The model under review builds one solid part; all positions refer to its coordinate system, in mm. A direction names the side the tool comes from. Coordinates: 2 decimals unless noted, no trailing zeros. Order: outer loops, then holes, each group sorted by start corner. A loop starts at its lowest first (then second) coordinate and runs counter-clockwise, first axis right, second up. Notation, with made-up numbers: (45.25, -2) - (72.25, -2) arc R7 cw to (72.25, 8) - close; hole circle Ø9 at (22, 42). An arc over 180 degrees is marked (long way). Answer in a Markdown table with one row per item.
```python
from build123d import *

# Parameters (mm, degrees)
F0_W     = 1620
F0_H     = 1350
F1_DEPTH = 525
F2_W     = 630
F2_H     = 540
F3_DEPTH = 420
F4_W     = 990
F4_H     = 450
F5_DEPTH = 540
F7_DEPTH = 1620.001
F9_DEPTH = 1050.001


with BuildPart() as f1:
    # F0 (on Front) → F1 (new body, symmetric)
    with BuildSketch(Plane.XZ):
        Rectangle(F0_W, F0_H)
    extrude(amount=F1_DEPTH, both=True)

    # F2 (on face) → F3 (cut)
    with BuildSketch(Plane.XZ.offset(525)):
        with Locations((-495, -405)):
            Rectangle(F2_W, F2_H)
        with Locations((495, -405)):
            Rectangle(F2_W, F2_H)
    extrude(amount=-F3_DEPTH, mode=Mode.SUBTRACT)

    # F4 (on face) → F5 (cut)
    with BuildSketch(Plane.XY.offset(675)):
        with Locations((-315, -300)):
            Rectangle(F4_W, F4_H)
    extrude(amount=-F5_DEPTH, mode=Mode.SUBTRACT)

    # F6 (on face) → F7 (cut, through all)
    with BuildSketch(Plane.YZ.offset(810)):
        Polygon((135, 675), (-525, 675), (-525, 135), align=None)
    extrude(amount=-F7_DEPTH, mode=Mode.SUBTRACT)

    # F8 (on face) → F9 (cut, through all)
    with BuildSketch(Plane.XZ.offset(525)):
        Polygon((180, 675), (810, 135), (810, 675), align=None)
    extrude(amount=-F9_DEPTH, mode=Mode.SUBTRACT)


solid = f1.part
```
Item 1: To check wall thickness, follow line 1 (X direction, y = -370.5, z = -157); line 2 (Y direction, x = 679, z = -582); line 3 (Y direction, x = -382, z = 205.5). State the ranges of each line that lie inside material, in increasing order. Write a range as from..to.
Check values:
| item | result |
|---|---|
| line 1 | -180..180 |
| line 2 | -105..525 |
| line 3 | -75..525 |
Item 2: We need section D-D, the plane x = 18. Write out the cut boundary in (y, z).
Check values:
| item | result |
|---|---|
| outline | (-525, -675) - (525, -675) - (525, 675) - (135, 675) - (-75, 503.18) - (-75, 135) - (-525, 135) - close |
Item 3: Clearance check with flat-ended pins moving along their axes: pin 1 Ø12 at (y, z) = (144, 455.5) entering from +X; pin 2 Ø1.5 at (y, z) = (343, 179.5) entering from +X; pin 3 Ø1 at (y, z) = (-161, 209) entering from -X. State where each tip first meets the part, or that it passes through.
Check values:
| item | result |
|---|---|
| pin 1 | x = 443.08 |
| pin 2 | x = 758.96 |
| pin 3 | x = 180 |
Item 4: We need section C-C, the plane y = -396.5. Write out the cut boundary in (x, z), then the cut area to 3 significant figures.
Check values:
| item | result |
|---|---|
| outline | (-810, -135) - (-180, -135) - (-180, -675) - (180, -675) - (180, -135) - (810, -135) - (810, 135) - (687.34, 240.14) - (180, 240.14) - (180, 135) - (-810, 135) - close |
| area | 692,000 mm^2 |
Item 5: We need section A-A, the plane x = -658.5. Write out the cut boundary in (y, z).
Check values:
| item | result |
|---|---|
| outline | (-525, -135) - (-105, -135) - (-105, -675) - (525, -675) - (525, 675) - (135, 675) - (-75, 503.18) - (-75, 135) - (-525, 135) - close |
Item 6: We need section B-B, the plane z = 198. Write out the cut boundary in (x, y), then the cut area to 3 significant figures.
Check values:
| item | result |
|---|---|
| outline | (-810, -75) - (180, -75) - (180, -448) - (736.5, -448) - (736.5, 525) - (-810, 525) - close |
| area | 1,140,000 mm^2 |
Item 7: Tool access review of faces 1 (the face through (180, -203, 240)), 2 (the face through (-322, 327, 675)), 3 (the face through (11.34, -52.953, 521.22)), 4 (the face through (491, -318, -135)), 5 (the face through (-499, -105, -401)): name each direction out of +Z, -Z, +X, -X, +Y, -Y from which nothing blocks a thin tool from reaching the whole face with its end or side.
Check values:
| item | result |
|---|---|
| face 1 | +Z, -X, -Y |
| face 2 | +Z, +X, -X, +Y, -Y |
| face 3 | +Z, +X, -X, -Y |
| face 4 | -Z, +X, -Y |
| face 5 | -Z, -X, -Y |
